Here's the drawing with two shaded views (mm, measured from the low corner). I have some questions. A direction names the side the tool comes from. Round coordinates to 2 decimals unless told otherwise and drop trailing zeros. Loops run counter-clockwise (first coordinate to the right, second up) from the corner with the lowest first, then second, coordinate; pieces in that order, holes last.
(1) If I drill on line 1 along Z through (x, y) = (5.5, 5.25); line 2 along Y through (x, z) = (3.75, 3); line 3 along Y through (x, z) = (1.5, 2.15), over which ranges is the centre line in solid material (lowest first)?
(2) Thinking about a two-plate mould opening in Z: for the marked faces 1, 2 and 3, which applies, released by +Z, released by -Z, zero draft, split by the parting line, or undercut?
(3) I want a section at C-C on x = 0.5. Write out the boundary of the cut face in (y, z), plus the area to 3 significant figures.
(4) I want a section at D-D on z = 3. Write out the boundary of the cut face in (x, y).
(5) I want a section at B-B on z = 1.8. Write out the boundary of the cut face in (x, y), plus the area to 3 significant figures.
(6) Which directions (+Z, -Z, +X, -X, +Y, -Y) give clear straight access to the entire face, cutting with the end or side of a thin tool? Please do the marked faces 4 and 5.
(7) I want a section at A-A on y = 7.75. Write out the boundary of the cut face in (x, z).
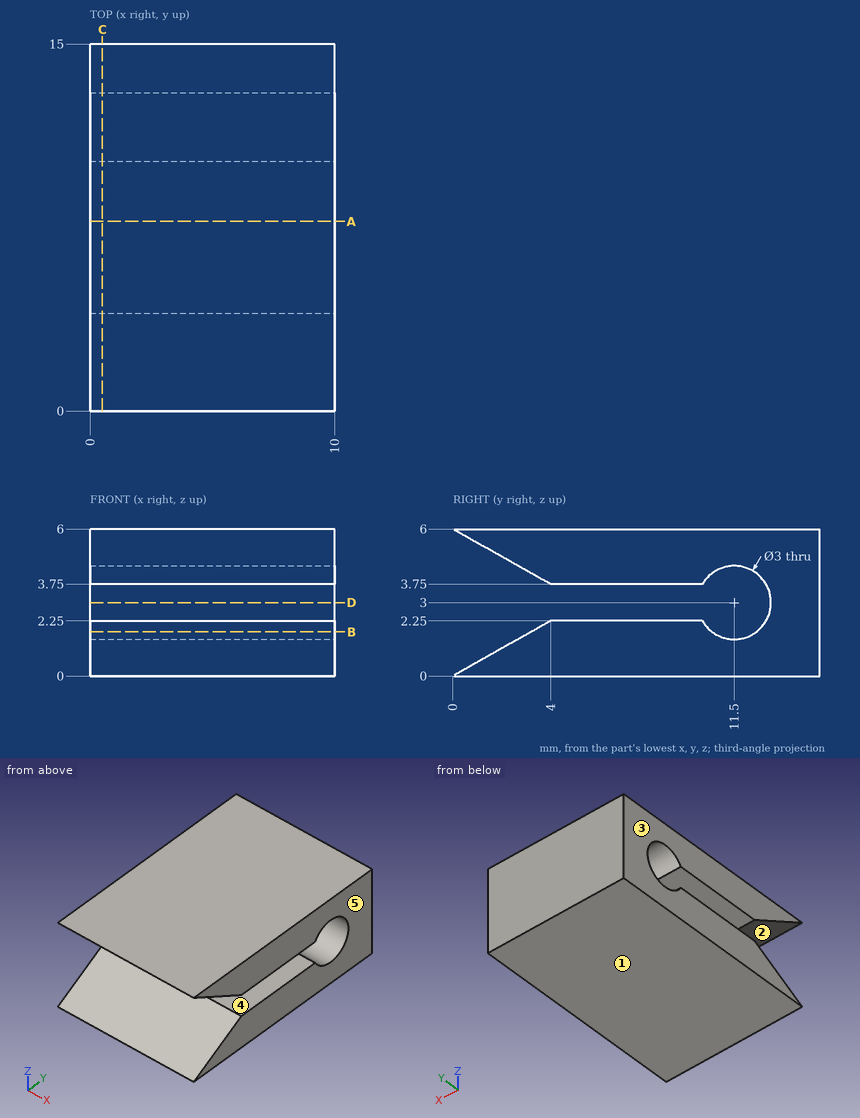
Filled sheet:
1. line 1: z = 0 to 2.25, 3.75 to 6
1. line 2: y = 13 to 15
1. line 3: y = 3.82 to 10.26, 12.74 to 15
2. face 1: released by -Z
2. face 2: undercut
2. face 3: zero draft
3. outline: (0, 0) - (15, 0) - (15, 6) - (0, 6) - (4, 3.75) - (10.2, 3.75) arc R1.5 cw (long way) to (10.2, 2.25) - (4, 2.25) - close
3. area: 58.8 mm2
4. outline: (0, 13) - (10, 13) - (10, 15) - (0, 15) - close
5. outline: (0, 3.2) - (10, 3.2) - (10, 10.6) - (0, 10.6) - close; (0, 12.4) - (10, 12.4) - (10, 15) - (0, 15) - close
5. area: 100 mm2
6. face 4: +X, -X, -Y
6. face 5: +Z, -Z, +X, +Y, -Y
7. outline: (0, 0) - (10, 0) - (10, 2.25) - (0, 2.25) - close; (0, 3.75) - (10, 3.75) - (10, 6) - (0, 6) - close
